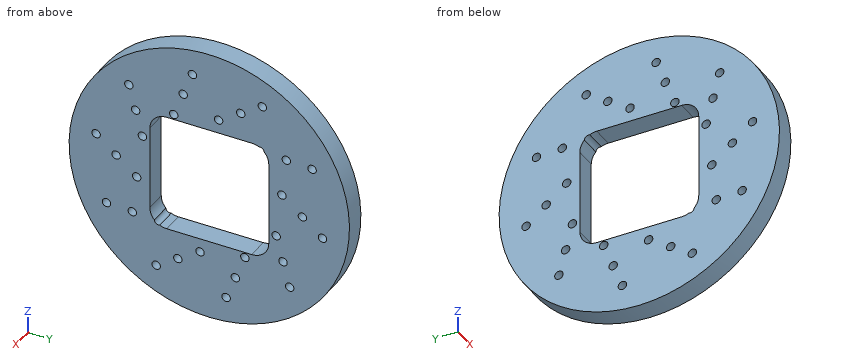
```python
from build123d import *

# Parameters (mm, degrees)
SKETCH1_R           = 16.5
BOSS_EXTRUDE1_DEPTH = 2.5
SKETCH2_W           = 14
SKETCH2_H           = 14
CUT_EXTRUDE2_DEPTH  = 2.5
FILLET1_R           = 2
SKETCH5_R           = 0.5
CUT_EXTRUDE3_DEPTH  = 2.5
CIRPATTERN3_COUNT   = 10


with BuildPart() as part:
    # Sketch1 → Boss-Extrude1 (new body)
    with BuildSketch(Plane(origin=(0, 0, 0), x_dir=(0, 0, -1), z_dir=(1, 0, 0))):
        Circle(SKETCH1_R)
    extrude(amount=BOSS_EXTRUDE1_DEPTH)

    # Sketch2 → Cut-Extrude2 (cut)
    with BuildSketch(Plane(origin=(2.5, 0, 0), x_dir=(0, 0, -1), z_dir=(1, 0, 0))):
        Rectangle(SKETCH2_W, SKETCH2_H)
    extrude(amount=-CUT_EXTRUDE2_DEPTH, mode=Mode.SUBTRACT)

    # Fillet1
    fillet1_edges = [part.edges().sort_by_distance(p)[0] for p in [
        (1.25, -7, -7),
        (1.25, -7, 7),
        (1.25, 7, 7),
        (1.25, 7, -7),
    ]]
    fillet(fillet1_edges, radius=FILLET1_R)

    # Sketch5 → Cut-Extrude3 (cut)
    with BuildSketch(Plane(origin=(2.5, 0, 0), x_dir=(0, 0, -1), z_dir=(1, 0, 0))):
        with Locations((-1.625921047, 8.546877008)):
            Circle(SKETCH5_R)
        with Locations((0.330939682, 10.964175556)):
            Circle(SKETCH5_R)
        with Locations((2.24289984, 13.326008692)):
            Circle(SKETCH5_R)
    cut_extrude3 = extrude(amount=-CUT_EXTRUDE3_DEPTH, mode=Mode.SUBTRACT)

    # CirPattern3: Cut-Extrude3 ×10 about axis
    cirpattern3_axis = Axis((0, 0, 0), (1, 0, 0))
    for i in range(1, CIRPATTERN3_COUNT):
        add(cut_extrude3.rotate(cirpattern3_axis, i * 360 / CIRPATTERN3_COUNT), mode=Mode.SUBTRACT)


solid = part.part
```
CAD build for the part. Positions are in the model's coordinates, mm. Give positions to 0.01 mm unless a question says otherwise; leave off trailing zeros. Loops run counter-clockwise (first coordinate to the right, second up) from the corner with the lowest first, then second, coordinate; pieces in that order, holes last. Notation, with made-up numbers: (14.25, 77.5) - (18.25, 77.5) arc R34 ccw to (18.25, 107.5) - close; hole circle Ø8 at (67.5, 33.25). An arc over 180 degrees is marked (long way). Put each result on its own line as item: value.
Q1. Slice it at A-A (y = 0). Give the cut face in (x, z), plus the area to 3 significant figures.
Filled in:
outline: (0, -16.5) - (2.5, -16.5) - (2.5, -7) - (0, -7) - close; (0, 7) - (2.5, 7) - (2.5, 16.5) - (0, 16.5) - close
area: 47.5 mm²
Q2. Probe line 1 along Y through (x, z) = (0.9, 2.5); line 2 along Y through (x, z) = (2.25, 4); line 3 along Z through (x, y) = (0.55, -4). List the from-to ranges inside material, lowest first.
Filled in:
line 1: y = -16.31 to -13.75, -12.9 to -7, 7 to 16.31
line 2: y = -16.01 to -8.28, -7.46 to -7, 7 to 16.01
line 3: z = -16.01 to -10.73, -9.92 to -7, 7 to 7.16, 8.09 to 16.01
Q3. Flat gauge pins, fed straight in: pin 1 (0.8 mm diameter, centred on x = 1.5, z = -1, fed in from -Y); pin 2 (1 mm diameter, centred on x = 2, z = -5.5, fed in from -Y); pin 3 (1.5 mm diameter, centred on x = 0.5, z = -6, fed in from +Y). Where does each tip first touch, or does it go through?
Filled in:
pin 1: stops at y = -16.49
pin 2: stops at y = -15.72
pin 3: stops at y = 15.64
Q4. Slice it at B-B (x = 0.6). Give the number of separate pieces and of enclosed holes in the cut face, plus the area to 3 significant figures.
Filled in:
separate pieces: 1
enclosed holes: 29
area: 641 mm²
